from build123d import *

# Parameters (mm, degrees)
F1_R           = 8.89
F1_R_2         = 5.969
F3_DEPTH       = 3.556
F5_R           = 8.89
F5_R_2         = 7.62
F7_DEPTH       = 3.556
F8_DEPTH       = 25.4
F8_DEPTH_BACK  = 25.4
F0_W           = 10.282781499
F0_H           = 12.7
F0_W_2         = 17.657218501
F11_DEPTH      = 8.89
F11_DEPTH_BACK = 8.89
F9_R           = 7.62
F10_R          = 7.62
F12_DEPTH      = 25.4


# Not quite as in the source:
# - a feature of the source that left no trace in its solid (it failed there, or was rolled back) is left out
# - a pattern or mirror of a feature is missing from the dataset's text; its kind, count and spacing are read off the source's solid


with BuildPart() as f2:
    # F2: sweep along a path in F0
    with BuildLine(Plane.XY) as f2_path:
        Line((0, 0), (0, 70.4088))
        ThreePointArc((0, 70.4088), (13.97, 84.3788), (27.94, 70.4088))
        Line((27.94, 70.4088), (27.94, 0))
        Line((27.94, 0), (27.94, -3.556))
    # F1 (on Front) → F2 (sweep)
    with BuildSketch(Plane.XZ):
        Circle(F1_R)
        Circle(F1_R_2, mode=Mode.SUBTRACT)
    sweep(path=f2_path.line)

    # F3 (add): a face of the model
    f3_faces = [f2.faces().sort_by_distance(p)[0] for p in [
        (-8.6385528286, 0, 0),
    ]]
    extrude(f3_faces, amount=F3_DEPTH)

    # F5 (on face) → F7 (cut)
    with BuildSketch(Plane.XZ.offset(3.556)):
        with Locations((27.94, 0)):
            Circle(F5_R)
        with Locations((27.94, 0)):
            Circle(F5_R_2, mode=Mode.SUBTRACT)
    f7 = extrude(amount=-F7_DEPTH, mode=Mode.SUBTRACT)

    # F7_copies: F7 across plane
    add(f7.mirror(Plane(origin=(13.97, 0, 0), x_dir=(0, 0, -1), z_dir=(-1, 0, 0))), mode=Mode.SUBTRACT)

    # F0 (on Top) → F8 (cut, two sides)
    with BuildSketch(Plane.XY) as f8_sk:
        with BuildLine():
            Line((-21.5208670124, 32.3088), (0, 32.3088))
            Line((0, 32.3088), (0, 70.4088))
            ThreePointArc((0, 70.4088), (13.97, 84.3788), (27.94, 70.4088))
            Line((27.94, 70.4088), (27.94, 32.3088))
            Line((27.94, 32.3088), (57.1982562542, 32.3088))
            Line((57.1982562542, 32.3088), (57.1982562542, 105.6616994024))
            Line((57.1982562542, 105.6616994024), (-21.5208670124, 105.6616994024))
            Line((-21.5208670124, 105.6616994024), (-21.5208670124, 32.3088))
        make_face()
        with BuildLine():
            Line((0, 70.4088), (0, 32.3088))
            Line((0, 32.3088), (13.97, 32.3088))
            Line((13.97, 32.3088), (27.94, 32.3088))
            Line((27.94, 32.3088), (27.94, 70.4088))
            ThreePointArc((27.94, 70.4088), (13.97, 84.3788), (0, 70.4088))
        make_face()
    extrude(amount=-F8_DEPTH, mode=Mode.SUBTRACT)
    extrude(f8_sk.sketch, amount=F8_DEPTH_BACK, mode=Mode.SUBTRACT)

    # F0 (on Top) → F11 (join, two sides)
    with BuildSketch(Plane.XY) as f11_sk:
        with Locations((22.7986092505, 17.9638495505)):
            Rectangle(F0_W, F0_H)
        with Locations((8.8286092505, 17.9638495505)):
            Rectangle(F0_W_2, F0_H)
    extrude(amount=F11_DEPTH)
    extrude(f11_sk.sketch, amount=-F11_DEPTH_BACK)

    # F9 (on face) + F10 (on face) → F12 (cut)
    with BuildSketch(Plane(origin=(0, 32.3088, 0), x_dir=(-1, 0, 0), z_dir=(0, 1, 0))):
        with Locations((-27.94, 0)):
            Circle(F9_R)
    with BuildSketch(Plane(origin=(0, 32.3088, 0), x_dir=(-1, 0, 0), z_dir=(0, 1, 0))):
        Circle(F10_R)
    extrude(amount=-F12_DEPTH, mode=Mode.SUBTRACT)


solid = f2.part
Can you work these out from the model? Positions are in its coordinate system, mm. A direction names the side the tool comes from. Round coordinates to 2 decimals unless told otherwise and drop trailing zeros. Loops run counter-clockwise (first coordinate to the right, second up) from the corner with the lowest first, then second, coordinate; pieces in that order, holes last. Notation, with made-up numbers: (56.5, -29) - (83.5, -29) arc R22 cw to (83.5, 1) - close; hole circle Ø3 at (57, -12.75). An arc over 180 degrees is marked (long way). Answer in a Markdown table with one row per item. Add a question column.
Q1. I want a section at B-B on x = -5. List the corners of the cut face in (y, z) for me.
Q2. For pin 1 Ø5.5 at (x, z) = (15, -2.5) entering from +Y; pin 2 Ø2 at (y, z) = (3.5, -4.5) entering from -X; pin 3 Ø8 at (y, z) = (6, -6) entering from +X, each with a flat end and sliding along its axis, tell me the tip position at first contact or that it passes through.
Q3. I want a section at C-C on y = 2. List the corners of the cut face in (x, z) for me, and give its area (3 significant figures).
Q4. I want a section at D-D on z = 0. Count the separate pieces of the cut face and the enclosed holes in it, and give its area (3 significant figures).
Q5. I want a section at A-A on y = 19.5. List the corners of the cut face in (x, z) for me.
Q6. We'd pull the mould along Z, two halves only. Please class faces 1 (the flat face through (14, 18, -8.89)), 2 (the cylindrical face through (35.553, 19.787, 0.335)), 3 (the flat face through (-7, 0, 4)), 4 (the cylindrical face through (36.82, 15.93, -0.39)): pulls with the +Z half, pulls with the -Z half, needs draft (parallel to the pull), parting line crosses it, or undercut.
Q7. I need wall thicknesses on L1, parallel to Z at x = 0, y = 20.5; L2, parallel to Z at x = 0, y = 1.5; L3, parallel to X at y = 20, z = 4. Which ranges of each line are inside material? Lowest first, please.
Q8. Which directions (+Z, -Z, +X, -X, +Y, -Y) give clear straight access to the entire face, cutting with the end or side of a thin tool? Please do faces 5 (the cylindrical face through (-8.88, 16.38, -0.39)), 6 (the cylindrical face through (22.247, 1.603, -1.793)), 7 (the cylindrical face through (1.65, -1.8, -7.44)), 8 (the flat face through (5, 6.909, -4)), 9 (the flat face through (32, 32.309, -7)).
A:
| question | item | result |
|---|---|---|
| 1 | outline | (-3.56, -5.75) - (0, -5.75) - (0, -7.35) - (32.31, -7.35) - (32.31, -5.75) - (6.91, -5.75) - (6.91, -3.26) - (-3.56, -3.26) - close; (-3.56, 3.26) - (6.91, 3.26) - (6.91, 5.75) - (32.31, 5.75) - (32.31, 7.35) - (0, 7.35) - (0, 5.75) - (-3.56, 5.75) - close |
| 2 | pin 1 | y = 24.31 |
| 2 | pin 2 | x = -8.17 |
| 2 | pin 3 | x = 36.6 |
| 3 | outline | circle Ø17.78 at (0, 0); circle Ø17.78 at (27.94, 0); hole circle Ø11.94 at (0, 0); hole circle Ø11.94 at (27.94, 0) |
| 3 | area | 273 mm^2 |
| 4 | separate pieces | 3 |
| 4 | enclosed holes | 0 |
| 4 | area | 362 mm^2 |
| 5 | outline | (0, -8.89) - (27.94, -8.89) arc R8.89 ccw to (27.94, 8.89) - (0, 8.89) arc R8.89 ccw to start; hole circle Ø15.24 at (0, 0); hole circle Ø15.24 at (27.94, 0) |
| 6 | face 1 | pulls with the -Z half |
| 6 | face 2 | undercut |
| 6 | face 3 | needs draft |
| 6 | face 4 | parting line crosses it |
| 7 | L1 | -8.89 to -7.62, 7.62 to 8.89 |
| 7 | L2 | -8.89 to -5.97, 5.97 to 8.89 |
| 7 | L3 | -7.94 to -6.49, 6.49 to 21.45, 34.43 to 35.88 |
| 8 | face 5 | none |
| 8 | face 6 | +Y, -Y |
| 8 | face 7 | -Y |
| 8 | face 8 | +Y |
| 8 | face 9 | +Z, -Z, +X, -X, +Y |
